```python
from build123d import *

# Parameters (mm, degrees)
SKETCH1_R           = 1.143
BOSS_EXTRUDE1_DEPTH = 1.524
SKETCH2_R           = 1.524
SKETCH2_R_2         = 1.143
CUT_EXTRUDE1_DEPTH  = 25.96925768
SKETCH4_R           = 20.695463349
SKETCH4_R_2         = 15.2527
CUT_EXTRUDE2_DEPTH  = 25.96925768
BOSS_EXTRUDE2_DEPTH = 3.048
BOSS_EXTRUDE3_DEPTH = 3.048


with BuildPart() as part:
    # Sketch1 → Boss-Extrude1 (new, symmetric)
    with BuildSketch(Plane(origin=(0, 0, 0), x_dir=(1, 0, 0), z_dir=(0, 1, 0))):
        with BuildLine():
            ThreePointArc((-17.060660873, -5.2832), (-0.126583546, -17.859516463), (16.984058744, -5.5245))
            Line((16.984058744, -5.5245), (16.984058744, 5.5245))
            ThreePointArc((16.984058744, 5.5245), (-0.338525345, 17.856756488), (-17.181244816, 4.8768))
            Line((-17.181244816, 4.8768), (-6.056265338, 4.8768))
            Line((-6.056265338, 4.8768), (-6.056265338, -5.2832))
            Line((-6.056265338, -5.2832), (-17.060660873, -5.2832))
        make_face()
        with Locations(Location((8.579035657, 10.1092, 0), (0, 0, 90))):
            Circle(SKETCH1_R, mode=Mode.SUBTRACT)
        with Locations(Location((0, -13.2588, 0), (0, 0, 90))):
            Circle(SKETCH1_R, mode=Mode.SUBTRACT)
        with Locations(Location((-10.832526773, -7.6454, 0), (0, 0, 90))):
            Circle(SKETCH1_R, mode=Mode.SUBTRACT)
        Polygon((6.036511594, -9.279669889), (4.875306175, -7.966959435), (1.641092014, -10.827900322), (2.802297432, -12.140610776), align=None, mode=Mode.SUBTRACT)
        Polygon((-5.027565338, -0.720652536), (-2.425370717, -3.662361234), (-8.720293025, -9.230761998), (-4.338426069, -14.184340812), (6.008776335, -5.031349407), (8.129238404, -7.428472845), (10.526361842, -5.308010776), (8.405899773, -2.910887338), (12.420130291, 0.640045174), (3.551213542, 10.666109075), (-0.463016976, 7.115176563), (-2.583479045, 9.5123), (-4.980602482, 7.391837931), (-2.860140414, 4.994714494), (-4.515281158, 3.5306), align=None, mode=Mode.SUBTRACT)
        Polygon((0.846775502, 8.816385505), (5.032229122, 12.518779594), (3.181032078, 14.611506404), (-1.004421543, 10.909112315), align=None, mode=Mode.SUBTRACT)
    extrude(amount=BOSS_EXTRUDE1_DEPTH, both=True)

    # Sketch2 → Cut-Extrude1 (cut, through all)
    # profile 1 of 6: a face of its own
    with BuildSketch(Plane(origin=(0, 1.524, 0), x_dir=(1, 0, 0), z_dir=(0, 1, 0))):
        with Locations((-10.832526773, -7.6454)):
            Circle(SKETCH2_R)
        with Locations((-10.832526773, -7.6454)):
            Circle(SKETCH2_R_2, mode=Mode.SUBTRACT)
    # profile 2 of 6: a face of its own
    with BuildSketch(Plane(origin=(0, 1.524, 0), x_dir=(1, 0, 0), z_dir=(0, 1, 0))):
        with BuildLine():
            ThreePointArc((-15.417270145, -9.015882261), (-14.591708872, -10.298562224), (-13.659706927, -11.506118301))
            Line((-13.659706927, -11.506118301), (-9.953745163, -8.89051802))
            ThreePointArc((-9.953745163, -8.89051802), (-12.077644792, -8.524181609), (-11.711308382, -6.40028198))
            Line((-11.711308382, -6.40028198), (-15.417270145, -9.015882261))
        make_face()
    # profile 3 of 6: a face of its own
    with BuildSketch(Plane(origin=(0, 1.524, 0), x_dir=(1, 0, 0), z_dir=(0, 1, 0))):
        with BuildLine():
            ThreePointArc((1.524, -13.2588), (0, -14.7828), (-1.524, -13.2588))
            Line((-1.524, -13.2588), (-1.524, -17.794824407))
            ThreePointArc((-1.524, -17.794824407), (0, -17.859965052), (1.524, -17.794824407))
            Line((1.524, -17.794824407), (1.524, -13.2588))
        make_face()
    # profile 4 of 6: a face of its own
    with BuildSketch(Plane(origin=(0, 1.524, 0), x_dir=(1, 0, 0), z_dir=(0, 1, 0))):
        with Locations((0, -13.2588)):
            Circle(SKETCH2_R)
        with Locations((0, -13.2588)):
            Circle(SKETCH2_R_2, mode=Mode.SUBTRACT)
    # profile 5 of 6: a face of its own
    with BuildSketch(Plane(origin=(0, 1.524, 0), x_dir=(1, 0, 0), z_dir=(0, 1, 0))):
        with BuildLine():
            Line((10.352068988, 14.55379742), (7.417058645, 11.095296053))
            ThreePointArc((7.417058645, 11.095296053), (9.104260863, 11.539834294), (10.103035657, 10.1092))
            ThreePointArc((10.103035657, 10.1092), (10.009669951, 9.583974794), (9.741012668, 9.123103947))
            Line((9.741012668, 9.123103947), (12.676023011, 12.581605315))
            ThreePointArc((12.676023011, 12.581605315), (11.556194906, 13.61736799), (10.352068988, 14.55379742))
        make_face()
    # profile 6 of 6: a face of its own
    with BuildSketch(Plane(origin=(0, 1.524, 0), x_dir=(1, 0, 0), z_dir=(0, 1, 0))):
        with Locations((8.579035657, 10.1092)):
            Circle(SKETCH2_R)
        with Locations((8.579035657, 10.1092)):
            Circle(SKETCH2_R_2, mode=Mode.SUBTRACT)
    extrude(amount=-CUT_EXTRUDE1_DEPTH, mode=Mode.SUBTRACT)

    # Sketch4 → Cut-Extrude2 (cut, through all)
    with BuildSketch(Plane(origin=(0, 1.524, 0), x_dir=(1, 0, 0), z_dir=(0, 1, 0))):
        Circle(SKETCH4_R)
        Circle(SKETCH4_R_2, mode=Mode.SUBTRACT)
    extrude(amount=-CUT_EXTRUDE2_DEPTH, mode=Mode.SUBTRACT)

    # Sketch5 → Boss-Extrude2 (add)
    with BuildSketch(Plane(origin=(0, 1.524, 0), x_dir=(1, 0, 0), z_dir=(0, 1, 0))):
        Polygon((-2.425370717, -3.662361234), (1.956496239, -8.615940048), (1.005256779, -9.45739325), (-3.376610176, -4.503814436), align=None)
    extrude(amount=-BOSS_EXTRUDE2_DEPTH)

    # Sketch6 → Boss-Extrude3 (add)
    with BuildSketch(Plane(origin=(0, 1.524, 0), x_dir=(1, 0, 0), z_dir=(0, 1, 0))):
        with BuildLine():
            Line((-11.711308382, -6.40028198), (-9.953745163, -8.89051802))
            ThreePointArc((-9.953745163, -8.89051802), (-9.587408753, -6.766618391), (-11.711308382, -6.40028198))
        make_face()
        with BuildLine():
            Line((-1.524, -13.2588), (1.524, -13.2588))
            ThreePointArc((1.524, -13.2588), (0, -11.7348), (-1.524, -13.2588))
        make_face()
        with BuildLine():
            Line((7.417058645, 11.095296053), (9.741012668, 9.123103947))
            ThreePointArc((9.741012668, 9.123103947), (7.592939604, 8.947222989), (7.417058645, 11.095296053))
        make_face()
        Polygon((4.353635591, -6.495463901), (0.071641066, -6.485163659), (1.956496239, -8.615940048), align=None)
    extrude(amount=-BOSS_EXTRUDE3_DEPTH)


solid = part.part
```
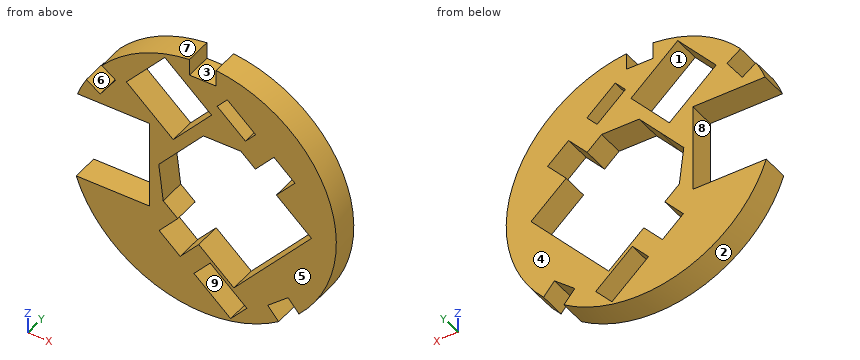
Build history of the part. All positions in model axes, mm. Face numbers are marked on the shaded views. A direction names the side the tool comes from. Round coordinates to 2 decimals unless told otherwise and drop trailing zeros. Write each loop counter-clockwise with the first axis right and the second up, starting at its lowest first coordinate (ties: lowest second). Pieces come first, ordered by that corner, then holes.
1) Drill centre lines: probe 1 along Z at (x, y) = (-7, 1.35); probe 2 along X at (y, z) = (1.25, 9.5); probe 3 along Z at (x, y) = (3.5, -1.4). Where is each one in solid material? Low to high.
2) Band-saw the part on A-A, the plane z = -6. List the corners of the cut face in (x, y), and give its area (3 significant figures).
3) Mould opens along Z. For the marked faces 1, 2, 3 and 4 say: +Z half, -Z half, draft (parallel to the pull), parting line (faces both ways), or undercut.
4) Band-saw the part on D-D, the plane y = -1. Give the number of separate pieces and of enclosed holes in the cut face, and give its area (3 significant figures).
5) Pin check, flat tips, straight feed: pin 1 (1.5 mm diameter, centred on x = -0.5, y = 0.5, fed in from +Z); pin 2 (0.6 mm diameter, centred on y = -0.5, z = 14, fed in from +X); pin 3 (1.5 mm diameter, centred on y = -0.5, z = -1.5, fed in from -X); pin 4 (2 mm diameter, centred on x = 4.5, z = 9, fed in from -Y). Stop position of each tip, or through.
6) Band-saw the part on B-B, the plane x = -7.5. List the corners of the cut face in (y, z).
7) Band-saw the part on C-C, the plane x = 6.5. List the corners of the cut face in (y, z).
8) 3-axis set-ups, long thin cutter, end or side, ignore diameter. For the marked faces 5, 6, 7, 8 and 9: which of +Z, -Z, +X, -X, +Y, -Y reach the whole face in a straight line?
Ans:
1. probe 1: z = -13.55 to -4.88, 5.28 to 7.71, 11.18 to 13.55
1. probe 2: x = -10.82 to -8.48, 0.96 to 3.14, 5.79 to 11.93
1. probe 3: z = -14.85 to -14.25, -11.16 to -10.62, 6.49 to 9.18, 11.52 to 14.85
2. outline: (-14.02, -1.52) - (-3.75, -1.52) - (-3.75, 1.52) - (-14.02, 1.52) - close; (7.68, -1.52) - (14.02, -1.52) - (14.02, 1.52) - (7.68, 1.52) - close
2. area: 50.7 mm2
3. face 1: undercut
3. face 2: -Z half
3. face 3: +Z half
3. face 4: draft
4. separate pieces: 1
4. enclosed holes: 4
4. area: 354 mm2
5. pin 1: stops at z = 13.26
5. pin 2: stops at x = 6.7
5. pin 3: stops at x = -6.06
5. pin 4: stops at y = -1.52
6. outline: (-1.52, -13.28) - (1.52, -13.28) - (1.52, -4.88) - (-1.52, -4.88) - close; (-1.52, 5.28) - (1.52, 5.28) - (1.52, 8.15) - (-1.52, 8.15) - close; (-1.52, 10.61) - (1.52, 10.61) - (1.52, 13.28) - (-1.52, 13.28) - close
7. outline: (-1.52, -13.8) - (1.52, -13.8) - (1.52, -7.33) - (-1.52, -7.33) - close; (-1.52, 5.59) - (1.52, 5.59) - (1.52, 13.8) - (-1.52, 13.8) - close
8. face 5: +Z, -Z, +X, -X, -Y
8. face 6: +Z, +Y, -Y
8. face 7: +Z, -X, +Y, -Y
8. face 8: -X, +Y, -Y
8. face 9: +Y, -Y
